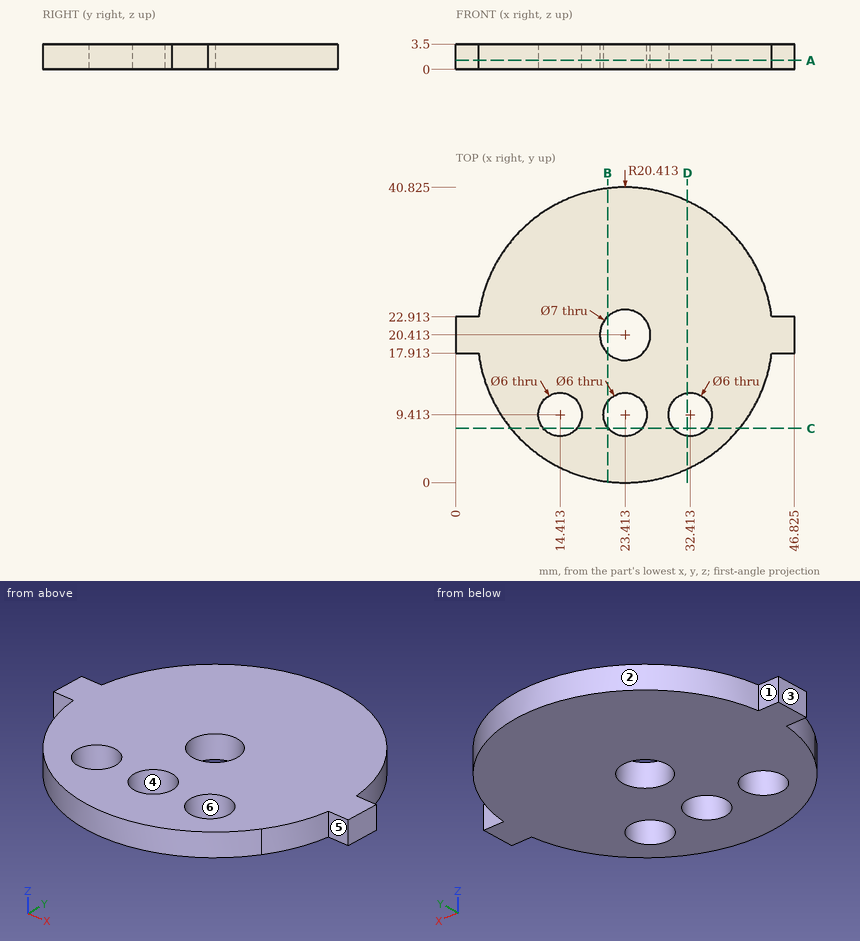
The drawing under review shows one solid part. Ordinate dimensions are in mm from its lowest x, y, z. A direction names the side the tool comes from. Round coordinates to 2 decimals unless told otherwise and drop trailing zeros. Order: outer loops, then holes, each group sorted by start corner. A loop starts at its lowest first (then second) coordinate and runs counter-clockwise, first axis right, second up. Notation, with made-up numbers: (42, -27.75) - (84, -27.75) arc R26 cw to (84, 9.25) - close; hole circle Ø11 at (20.5, 10). An arc over 180 degrees is marked (long way). Return JSON: item names as keys, results as strings.
Q1. Consider section C-C on y = 7.5. Write out the cut boundary in (x, z).
Computed values:
{"outline": "(7.6, 0) - (12.1, 0) - (12.1, 3.5) - (7.6, 3.5) - close; (16.72, 0) - (21.1, 0) - (21.1, 3.5) - (16.72, 3.5) - close; (25.72, 0) - (30.1, 0) - (30.1, 3.5) - (25.72, 3.5) - close; (34.72, 0) - (39.22, 0) - (39.22, 3.5) - (34.72, 3.5) - close"}
Q2. Machinability: for the marked faces 1 and 2, which of the approach directions +Z, -Z, +X, -X, +Y, -Y give a long, thin tool a straight path to every point of the face, cutting with its end or side? Answer none if there is none.
Computed values:
{"face 1": "+Z, -Z, -X, +Y", "face 2": "+Z, -Z, +Y"}
Q3. Consider section D-D on x = 32. Write out the cut boundary in (y, z) (1 decimal), plus the area to 3 significant figures.
Computed values:
{"outline": "(1.9, 0) - (6.4, 0) - (6.4, 3.5) - (1.9, 3.5) - close; (12.4, 0) - (38.9, 0) - (38.9, 3.5) - (12.4, 3.5) - close", "area": "109 mm2"}
Q4. The part is to be moulded in two halves that separate along X. For the marked faces 3, 4, 5 and 6, say which applies: pulls with the +X half, pulls with the -X half, needs draft (parallel to the pull), parting line crosses it, or undercut.
Computed values:
{"face 3": "pulls with the -X half", "face 4": "undercut", "face 5": "needs draft", "face 6": "undercut"}
Q5. Wall thickness on L1, parallel to X at y = 12, z = 2.9 (1 decimal); L2, parallel to Y at x = 25.5, z = 1.4 (1 decimal); L3, parallel to X at y = 10, z = 2.55 (1 decimal): over which ranges is each line inside the solid? List them lowest first. Write a range as [from, to].
Computed values:
{"L1": "x = [4.8, 12.9], [15.9, 21.9], [24.9, 30.9], [33.9, 42]", "L2": "y = [0.1, 7.3], [11.6, 17.6], [23.2, 40.7]", "L3": "x = [5.9, 11.5], [17.4, 20.5], [26.4, 29.5], [35.4, 41]"}
Q6. Consider section B-B on x = 21. Write out the cut boundary in (y, z) (1 decimal).
Computed values:
{"outline": "(0.1, 0) - (7.6, 0) - (7.6, 3.5) - (0.1, 3.5) - close; (11.2, 0) - (17.9, 0) - (17.9, 3.5) - (11.2, 3.5) - close; (22.9, 0) - (40.7, 0) - (40.7, 3.5) - (22.9, 3.5) - close"}
Q7. Consider section A-A on z = 1.25. Write out the cut boundary in (x, y) (1 decimal).
Computed values:
{"outline": "(0, 17.9) - (3.2, 17.9) arc R20.4 ccw to (6.2, 9.4) arc R20.4 ccw to (40.6, 9.4) arc R20.4 ccw to (43.7, 17.9) - (46.8, 17.9) - (46.8, 22.9) - (43.7, 22.9) arc R20.4 ccw to (3.2, 22.9) - (0, 22.9) - close; hole circle Ø6 at (14.4, 9.4); hole circle Ø7 at (23.4, 20.4); hole circle Ø6 at (23.4, 9.4); hole circle Ø6 at (32.4, 9.4)"}
Q8. For pin 1 Ø1 at (y, z) = (27, 3) entering from +X; pin 2 Ø4 at (x, y) = (23.41, 20.41) entering from +Z; pin 3 Ø1.5 at (y, z) = (23.5, 3) entering from +X (1 decimal), all flat-tipped, find the tip position at first contact; note any pin that passes through.
Computed values:
{"pin 1": "stops at x = 42.9", "pin 2": "passes through", "pin 3": "stops at x = 46.8"}
